Geometry: final body of the model. Coordinates: model frame, mm. A direction names the side the tool comes from. Coordinates: 2 decimals unless noted, no trailing zeros. Order: outer loops, then holes, each group sorted by start corner. A loop starts at its lowest first (then second) coordinate and runs counter-clockwise, first axis right, second up. Notation, with made-up numbers: (-27, -39.5) -> (7, -39.5) arc R8 ccw to (7, -26.5) -> close; hole circle Ø10 at (8, 35.25). An arc over 180 degrees is marked (long way). Use one line per item in the form item = value.
```python
from build123d import *

# Parameters (mm, degrees)
SKETCH_1_R          = 2.5
EXTRUDE_1_DEPTH     = 30
CUT_EXTRUDE_1_REACH = 37.984
SKETCH_2_R          = 2
FILLET_1_R          = 1
SKETCH_3_R          = 3.55
EXTRUDE_2_DEPTH     = 1


with BuildPart() as part:
    # 草图1 → 凸台-拉伸1 (new body)
    with BuildSketch(Plane(origin=(0, 0, 0), x_dir=(1, 0, 0), z_dir=(0, 1, 0))):
        with BuildLine():
            Line((19.464101615, -0.5), (3.464101615, -0.5))
            ThreePointArc((3.464101615, -0.5), (-3.5, 0), (3.464101615, 0.5))
            Line((3.464101615, 0.5), (19.464101615, 0.5))
            Line((19.464101615, 0.5), (19.464101615, -0.5))
        make_face()
        with Locations(Location((0, 0, 0), (0, 0, 270))):
            Circle(SKETCH_1_R, mode=Mode.SUBTRACT)
    extrude(amount=EXTRUDE_1_DEPTH)

    # 草图2 → 切除-拉伸1 (cut, up to next)
    with BuildSketch(Plane.XY.offset(0.5), mode=Mode.PRIVATE) as cut_extrude_1_sk1:
        with Locations((14.464101615, 24)):
            Circle(SKETCH_2_R)
    cut_extrude_1_tool1 = extrude(cut_extrude_1_sk1.sketch, amount=-CUT_EXTRUDE_1_REACH, mode=Mode.PRIVATE) & part.part
    # 草图2 → 切除-拉伸1 (cut, up to next)
    with BuildSketch(Plane.XY.offset(0.5), mode=Mode.PRIVATE) as cut_extrude_1_sk2:
        with Locations((8.139546295, 15)):
            Circle(SKETCH_2_R)
    cut_extrude_1_tool2 = extrude(cut_extrude_1_sk2.sketch, amount=-CUT_EXTRUDE_1_REACH, mode=Mode.PRIVATE) & part.part
    # 草图2 → 切除-拉伸1 (cut, up to next)
    with BuildSketch(Plane.XY.offset(0.5), mode=Mode.PRIVATE) as cut_extrude_1_sk3:
        with Locations((14.464101615, 6)):
            Circle(SKETCH_2_R)
    cut_extrude_1_tool3 = extrude(cut_extrude_1_sk3.sketch, amount=-CUT_EXTRUDE_1_REACH, mode=Mode.PRIVATE) & part.part
    add(cut_extrude_1_tool1.solids().sort_by_distance((14.464102, 24, 0.5))[0], mode=Mode.SUBTRACT)
    add(cut_extrude_1_tool2.solids().sort_by_distance((8.139546, 15, 0.5))[0], mode=Mode.SUBTRACT)
    add(cut_extrude_1_tool3.solids().sort_by_distance((14.464102, 6, 0.5))[0], mode=Mode.SUBTRACT)

    # 圆角1
    fillet_1_edges = [part.edges().sort_by_distance(p)[0] for p in [
        (19.464101615, 30, 0),
        (19.464101615, 0, 0),
    ]]
    fillet(fillet_1_edges, radius=FILLET_1_R)

    # 草图3 → 凸台-拉伸2 (add)
    with BuildSketch(Plane(origin=(0, 30, 0), x_dir=(1, 0, 0), z_dir=(0, 1, 0))):
        with Locations(Location((0, 0, 0), (0, 0, 8.09674977))):
            Circle(SKETCH_3_R)
    extrude(amount=EXTRUDE_2_DEPTH)


solid = part.part
```
1) Contact query for flat-ended pins moving along their axis: P1, Ø8, axis at x = 5.5, y = 5.5, coming from the +Z side; P2, Ø3, axis at x = 14.46, y = 6, coming from the +Z side; P3, Ø2, axis at x = 1.5, z = 1, coming from the -Y side; P4, Ø5, axis at x = 10, y = 20.5, coming from the +Z side. Output: stop coordinate, or through.
Results found:
P1 = 3.16
P2 = through
P3 = 0
P4 = 0.5
2) Access query for faces 1 (the cylindrical face through (-2.44, 14.79, -0.54)), 2 (the cylindrical face through (19.18, 29.7, 0.01)). Directions: +Z, -Z, +X, -X, +Y, -Y. A direction counts if a zero-diameter tool reaches every point of the face in a straight line with its end or side. Return the directions, or none.
Results found:
face_1 = -Y
face_2 = +Z, -Z, +X, +Y
3) Section A-A, the plane y = 15. Output: boundary loops of the cut face in (x, z).
Results found:
outline = (3.46, -0.5) -> (6.14, -0.5) -> (6.14, 0.5) -> (3.46, 0.5) arc R3.5 ccw (long way) to start; (10.14, -0.5) -> (19.46, -0.5) -> (19.46, 0.5) -> (10.14, 0.5) -> close; hole circle Ø5 at (0, 0)
4) Material intervals for probe 1 along Z at (x, y) = (10.75, 22); probe 2 along Z at (x, y) = (-0.5, 28); probe 3 along Y at (x, z) = (-0.75, 1.5), sorted ascending. Write a range as from..to.
Results found:
probe_1 = -0.5..0.5
probe_2 = -3.46..-2.45, 2.45..3.46
probe_3 = 30..31
5) Section B-B, the plane z = 0. Output: boundary loops of the cut face in (x, y), and give its area (3 significant figures).
Results found:
outline = (-3.55, 30) -> (-3.5, 30) -> (-3.5, 0) -> (-2.5, 0) -> (-2.5, 30) -> (2.5, 30) -> (2.5, 0) -> (18.46, 0) arc R1 ccw to (19.46, 1) -> (19.46, 29) arc R1 ccw to (18.46, 30) -> (3.55, 30) -> (3.55, 31) -> (-3.55, 31) -> close; hole circle Ø4 at (8.14, 15); hole circle Ø4 at (14.46, 6); hole circle Ø4 at (14.46, 24)
area = 508 mm2
6) Section D-D, the plane x = 7.75. Output: boundary loops of the cut face in (y, z).
Results found:
outline = (0, -0.5) -> (13.04, -0.5) -> (13.04, 0.5) -> (0, 0.5) -> close; (16.96, -0.5) -> (30, -0.5) -> (30, 0.5) -> (16.96, 0.5) -> close
7) Pull-direction query (Y, two-part tool) for faces 3 (the flat face through (11, 30, 0)), 4 (the cylindrical face through (9.21, 16.69, 0.01)), 5 (the flat face through (12, 15, 0.5)); classes: released by +Y, released by -Y, zero draft, split by the parting line, or undercut.
Results found:
face_3 = released by +Y
face_4 = undercut
face_5 = zero draft
8) Section C-C, the plane x = 15. Output: boundary loops of the cut face in (y, z).
Results found:
outline = (0, -0.5) -> (4.07, -0.5) -> (4.07, 0.5) -> (0, 0.5) -> close; (7.93, -0.5) -> (22.07, -0.5) -> (22.07, 0.5) -> (7.93, 0.5) -> close; (25.93, -0.5) -> (30, -0.5) -> (30, 0.5) -> (25.93, 0.5) -> close
